Check sheet for the modelled part. Datum: model origin and axes. Units: mm. A direction names the side the tool comes from. Give positions to 0.01 mm unless a question says otherwise; leave off trailing zeros. Order: outer loops, then holes, each group sorted by start corner. A loop starts at its lowest first (then second) coordinate and runs counter-clockwise, first axis right, second up.
Autodesk Fusion 360 part; units mm, degrees
sketch "Esquisse2" plane through (0, 0, 0) normal (0, 0, 1) x (1, 0, 0)
  line L0 (160, 106.25) -> (-160, 106.25)
  line L1 (-160, 106.25) -> (-160, -106.25)
  line L2 (160, -106.25) -> (160, 106.25)
  line L3 (160, 106.25) -> (-160, -106.25) construction
  line L4 (-160, 106.25) -> (160, -106.25) construction
  line L5 (0, 0) -> (65, 0) construction
  line L6 (95, 45) -> (65, 45)
  line L7 (65, 45) -> (65, -45)
  line L8 (65, -45) -> (95, -45)
  line L9 (95, -45) -> (95, 45)
  line L10 (95, 45) -> (65, -45) construction
  line L11 (65, 45) -> (95, -45) construction
  line L12 (110, 45) -> (95, 45)
  line L13 (95, 45) -> (95, -45)
  line L14 (95, -45) -> (110, -45)
  line L15 (110, -45) -> (110, 45)
  line L16 (110, 45) -> (95, -45) construction
  line L17 (95, 45) -> (110, -45) construction
  circle A0 centre (150, 96.25) radius 2.5
  line L18 (0, 2.5) -> (0, 20)
  circle A1 centre (-150, 96.25) radius 2.5
  circle A2 centre (150, -96.25) radius 2.5
  circle A3 centre (-150, -96.25) radius 2.5
  circle A4 centre (0, 86.25) radius 12.5
  circle A5 centre (115, -106.25) radius 12.5
  line L19 (0, 1.75) -> (0, 22.5)
  circle A6 centre (-115, -106.25) radius 12.5
  arc A7 (-131.5, -106.25) -> (-98.5, -106.25) centre (-115, -106.25) ccw
  line L20 (-160, -106.25) -> (-131.5, -106.25)
  arc A8 (98.5, -106.25) -> (131.5, -106.25) centre (115, -106.25) ccw
  line L21 (-98.5, -106.25) -> (98.5, -106.25)
  line L22 (131.5, -106.25) -> (160, -106.25)
  line L23 (-65, 45) -> (-65, -45)
  line L24 (-95, 45) -> (-65, 45)
  line L25 (-110, 45) -> (-95, 45)
  line L26 (-110, -45) -> (-110, 45)
  line L27 (-95, -45) -> (-110, -45)
  line L28 (-65, -45) -> (-95, -45)
  line L29 (-155, 70) -> (-150, 70)
  line L30 (-150, 70) -> (-150, 30)
  line L31 (-150, 30) -> (-155, 30)
  line L32 (-155, 30) -> (-155, 70)
  line L33 (-155, -30) -> (-155, -70)
  line L34 (-150, -30) -> (-155, -30)
  line L35 (-150, -70) -> (-150, -30)
  line L36 (-155, -70) -> (-150, -70)
  line L37 (150, -70) -> (150, -30)
  line L38 (155, -70) -> (150, -70)
  line L39 (155, -30) -> (155, -70)
  line L40 (150, -30) -> (155, -30)
  line L41 (155, 30) -> (155, 70)
  line L42 (155, 70) -> (150, 70)
  line L43 (150, 70) -> (150, 30)
  line L44 (150, 30) -> (155, 30)
  point P0 (80, 0)
  point P1 (102.5, 0)
  dimension "d39" = 212.5
  dimension "d40" = 65
  dimension "d41" = 50
  dimension "d42" = 30
  dimension "d43" = 15
  dimension "d44" = 90
  dimension "d45" = 90
  dimension "d46" = 5
  dimension "d47" = 10
  dimension "d48" = 10
  dimension "d49" = 25
  dimension "d50" = 20
  dimension "d51" = 25
  dimension "d52" = 45
  dimension "d54" = 4
  dimension "d56" = 4
  dimension "d57" = 28.5
  dimension "d58" = 5
  dimension "d59" = 40
  dimension "d60" = 5
  dimension "d61" = 30
extrude "Extrusion1" add sketch "Esquisse2" along normal blind 3
fillet "Congé1" radius 10 4 edges at (160, -106.25, 1.5) (-160, -106.25, 1.5) (-160, 106.25, 1.5) (160, 106.25, 1.5)
fillet "Congé2" radius 10 4 edges at (131.5, -106.25, 1.5) (98.5, -106.25, 1.5) (-131.5, -106.25, 1.5) (-98.5, -106.25, 1.5)
equation "baseWidth = 250 mm"
equation "baseDepth = ( maxPerimeter - sparePerimeter - 2 * baseWidth ) / 2"
equation "maxPerimeter = ( 2050 / 2 ) * 1 mm"
equation "maxDeployedPerimeter = ( 2200 / 2 ) * 1 mm"
equation "sparePerimeter = 100 mm"
equation "baseThickness = 3 mm"
equation "chamferWidth = 30 mm"
equation "motorLength = 65 mm"
equation "wheelHoleWidth = 30 mm"
equation "encoderWheelHoleWidth = 15 mm"
equation "encoderAndSupportWidth = 40 mm"
equation "d39 = baseDepth"
equation "d42 = wheelHoleWidth"
equation "d43 = encoderWheelHoleWidth"
equation "d45 = d44"
equation "d51 = d49"
(1) Set-up check for faces 4 (the face through (96.11, -108, 1.52)), 5 (the face through (157.15, 103.24, 1.52)): record each of +Z, -Z, +X, -X, +Y, -Y from which the full face is reachable in a straight line by a thin tool's end or side.
Response values:
face 4: +Z, -Z, -Y
face 5: +Z, -Z, +X, +Y
(2) Material ranges on L1, parallel to X at y = -35.5, z = 1.65; L2, parallel to X at y = 49.5, z = 0.45; L3, parallel to Y at x = -115, z = 1, recorded low to high.
Response values:
L1: x = -160 to -155, -150 to -110, -65 to 65, 110 to 150, 155 to 160
L2: x = -160 to -155, -150 to 150, 155 to 160
L3: y = -122.75 to -118.75, -93.75 to 106.25
(3) Cross-section at A-A on x = 115. Enter the section's corners in (y, z).
Response values:
outline: (-122.75, 0) - (-118.75, 0) - (-118.75, 3) - (-122.75, 3) - close; (-93.75, 0) - (106.25, 0) - (106.25, 3) - (-93.75, 3) - close
(4) Cross-section at B-B on y = 55. Enter the section's corners in (x, z), then the cut area to 3 significant figures.
Response values:
outline: (-160, 0) - (-155, 0) - (-155, 3) - (-160, 3) - close; (-150, 0) - (150, 0) - (150, 3) - (-150, 3) - close; (155, 0) - (160, 0) - (160, 3) - (155, 3) - close
area: 930 mm2
(5) Release check for a two-part mould opening along Y. For faces 1 (the face through (134.03, -107.905, 1.521)), 2 (the face through (-2, -7, 0)), 3 (the face through (-103.077, -110.005, 1.479)) record: released by +Y, released by -Y, zero draft, split by the parting line, or undercut.
Response values:
face 1: released by -Y
face 2: zero draft
face 3: undercut
(6) Cross-section at D-D on x = 0. Enter the section's corners in (y, z), then the cut area to 4 significant figures.
Response values:
outline: (-106.25, 0) - (73.75, 0) - (73.75, 3) - (-106.25, 3) - close; (98.75, 0) - (106.25, 0) - (106.25, 3) - (98.75, 3) - close
area: 562.5 mm2
(7) Cross-section at C-C on y = -33.5. Enter the section's corners in (x, z).
Response values:
outline: (-160, 0) - (-155, 0) - (-155, 3) - (-160, 3) - close; (-150, 0) - (-110, 0) - (-110, 3) - (-150, 3) - close; (-65, 0) - (65, 0) - (65, 3) - (-65, 3) - close; (110, 0) - (150, 0) - (150, 3) - (110, 3) - close; (155, 0) - (160, 0) - (160, 3) - (155, 3) - close
(8) Gauge pin test, flat ends, axial feed: pin 1 Ø2 at (x, y) = (53.5, 71.5) entering from -Z; pin 2 Ø1.5 at (x, z) = (145.5, 1.5) entering from -Y; pin 3 Ø0.9 at (x, z) = (152.5, 2) entering from +Y; pin 4 Ø15 at (x, y) = (115, -106.25) entering from -Z. Record the tip position at first contact, or that the pin passes through.
Response values:
pin 1: stops at z = 0
pin 2: stops at y = -106.25
pin 3: stops at y = 106.04
pin 4: passes through
